```python
from build123d import *

# Parameters (mm, degrees)
SKETCH_1_R          = 2.85
EXTRUDE_1_DEPTH     = 1
EXTRUDE_2_DEPTH     = 6
SKETCH_3_R          = 3.25
EXTRUDE_3_DEPTH     = 2
CHAMFER_3_SIZE      = 0.2
FILLET_2_R          = 0.3
CHAMFER_4_SIZE      = 0.2
CHAMFER_5_SIZE      = 0.3
SKETCH_5_R          = 2.7
CUT_EXTRUDE_1_DEPTH = 5
SKETCH_6_R          = 4
EXTRUDE_4_DEPTH     = 38
FILLET_3_R          = 2
CHAMFER_6_SIZE      = 0.5
SKETCH_7_W          = 4
SKETCH_7_H          = 1
CHAMFER_7_SIZE      = 0.1


with BuildPart() as part:
    # 草图1 → 凸台-拉伸1 (new body)
    with BuildSketch(Plane(origin=(0, 0, 0), x_dir=(1, 0, 0), z_dir=(0, 1, 0))):
        with Locations(Location((0, 0, 0), (0, 0, 270))):
            Circle(SKETCH_1_R)
    extrude(amount=EXTRUDE_1_DEPTH)

    # 草图2 → 凸台-拉伸2 (add)
    with BuildSketch(Plane(origin=(0, 1, 0), x_dir=(1, 0, 0), z_dir=(0, 1, 0))):
        Polygon((4.618802154, 0), (2.309401077, 4), (-2.309401077, 4), (-4.618802154, 0), (-2.309401077, -4), (2.309401077, -4), align=None)
    extrude(amount=EXTRUDE_2_DEPTH)

    # 草图3 → 凸台-拉伸3 (add)
    with BuildSketch(Plane(origin=(0, 7, 0), x_dir=(1, 0, 0), z_dir=(0, 1, 0))):
        with Locations(Location((0, 0, 0), (0, 0, 270))):
            Circle(SKETCH_3_R)
    extrude(amount=EXTRUDE_3_DEPTH)

    # 倒角3
    chamfer_3_edges = [part.edges().sort_by_distance(p)[0] for p in [
        (0, 1, -2.85),
        (3.464101615, 1, 2),
        (3.464101615, 1, -2),
        (0, 1, -4),
        (-3.464101615, 1, -2),
        (-3.464101615, 1, 2),
        (0, 1, 4),
    ]]
    chamfer(chamfer_3_edges, length=CHAMFER_3_SIZE)

    # 圆角2
    fillet_2_edges = [part.edges().sort_by_distance(p)[0] for p in [
        (0, 7, -3.25),
        (3.464101615, 7, 2),
        (3.464101615, 7, -2),
        (0, 7, -4),
        (-3.464101615, 7, -2),
        (-3.464101615, 7, 2),
        (0, 7, 4),
    ]]
    fillet(fillet_2_edges, radius=FILLET_2_R)

    # 倒角4
    chamfer_4_edges = [part.edges().sort_by_distance(p)[0] for p in [
        (0, 9, -3.25),
    ]]
    chamfer(chamfer_4_edges, length=CHAMFER_4_SIZE)

    # 倒角5
    chamfer_5_edges = [part.edges().sort_by_distance(p)[0] for p in [
        (0, 0, -2.85),
    ]]
    chamfer(chamfer_5_edges, length=CHAMFER_5_SIZE)

    # 草图5 → 切除-拉伸1 (cut)
    with BuildSketch(Plane(origin=(0, 9, 0), x_dir=(1, 0, 0), z_dir=(0, 1, 0))):
        with Locations(Location((0, 0, 0), (0, 0, 270))):
            Circle(SKETCH_5_R)
    extrude(amount=-CUT_EXTRUDE_1_DEPTH, mode=Mode.SUBTRACT)

    # 草图6 → 凸台-拉伸4 (add)
    with BuildSketch(Plane.XZ):
        with Locations(Location((0, 0, 0), (0, 0, 270))):
            Circle(SKETCH_6_R)
    extrude(amount=EXTRUDE_4_DEPTH)

    # 圆角3
    fillet_3_edges = [part.edges().sort_by_distance(p)[0] for p in [
        (0, -38, 4),
    ]]
    fillet(fillet_3_edges, radius=FILLET_3_R)

    # 倒角6
    chamfer_6_edges = [part.edges().sort_by_distance(p)[0] for p in [
        (0, 0, 4),
    ]]
    chamfer(chamfer_6_edges, length=CHAMFER_6_SIZE)

    # 草图7 → 切除-旋转1 (revolve, cut)
    with BuildSketch(Plane(origin=(0, 0, 0), x_dir=(0, 0, -1), z_dir=(1, 0, 0))):
        with Locations((-5.7, -32.5)):
            Rectangle(SKETCH_7_W, SKETCH_7_H)
        with Locations((-5.7, -29.5)):
            Rectangle(SKETCH_7_W, SKETCH_7_H)
    revolve(axis=Axis((0, 0, 0), (0, -1, 0)), mode=Mode.SUBTRACT)

    # 倒角7
    chamfer_7_edges = [part.edges().sort_by_distance(p)[0] for p in [
        (0, -33, 4),
        (0, -32, 4),
        (0, -30, 4),
        (0, -29, 4),
    ]]
    chamfer(chamfer_7_edges, length=CHAMFER_7_SIZE)


solid = part.part
```
For this review, take the finished solid that the model builds, in its own axes (mm). A direction names the side the tool comes from. Round coordinates to 2 decimals unless told otherwise and drop trailing zeros. Loops run counter-clockwise (first coordinate to the right, second up) from the corner with the lowest first, then second, coordinate; pieces in that order, holes last.
Q1. Insertion check: pin 1 Ø3 at (y, z) = (-9.5, -1) entering from -X; pin 2 Ø3 at (x, y) = (-3, -28.5) entering from -Z. Each pin has a flat end and moves straight along its axis. Give the tip position at first contact, or say it passes through.
Result sheet:
pin 1: stops at x = -4
pin 2: stops at z = -3.71
Q2. Mouldability with a two-part tool opening along Y and no side actions: class faces 4 (the face through (-1.978, 8.04, -2.579)), 5 (the face through (3.406, 6.91, 1.929)), 6 (the face through (3.612, -29.493, -0.802)) as +Y half, -Y half, draft (parallel to the pull), parting line (faces both ways), or undercut.
Result sheet:
face 4: draft
face 5: +Y half
face 6: undercut
Q3. To check wall thickness, follow line 1 along X through (y, z) = (7.75, 0); line 2 along Y through (x, z) = (-1.5, -3.5); line 3 along Y through (x, z) = (-2, 3). State the ranges of each line that lie inside material, in increasing order.
Result sheet:
line 1: x = -3.25 to -2.7, 2.7 to 3.25
line 2: y = -36.86 to -33, -32 to -30, -29 to -0.31, 1 to 7
line 3: y = -37.19 to -0.11, 1 to 7
Q4. Machinability: for faces 1 (the face through (-3.905, -34.53, 0.867)), 2 (the face through (3, 1, 2)), 3 (the face through (3.37, 6.91, -1.99)), which of the approach directions +Z, -Z, +X, -X, +Y, -Y give a long, thin tool a straight path to every point of the face, cutting with its end or side? Answer none if there is none.
Result sheet:
face 1: -Y
face 2: none
face 3: -Z, +X, +Y
Q5. Add section A-A on y = -24. Write out the cut boundary in (x, z).
Result sheet:
outline: circle Ø8 at (0, 0)
